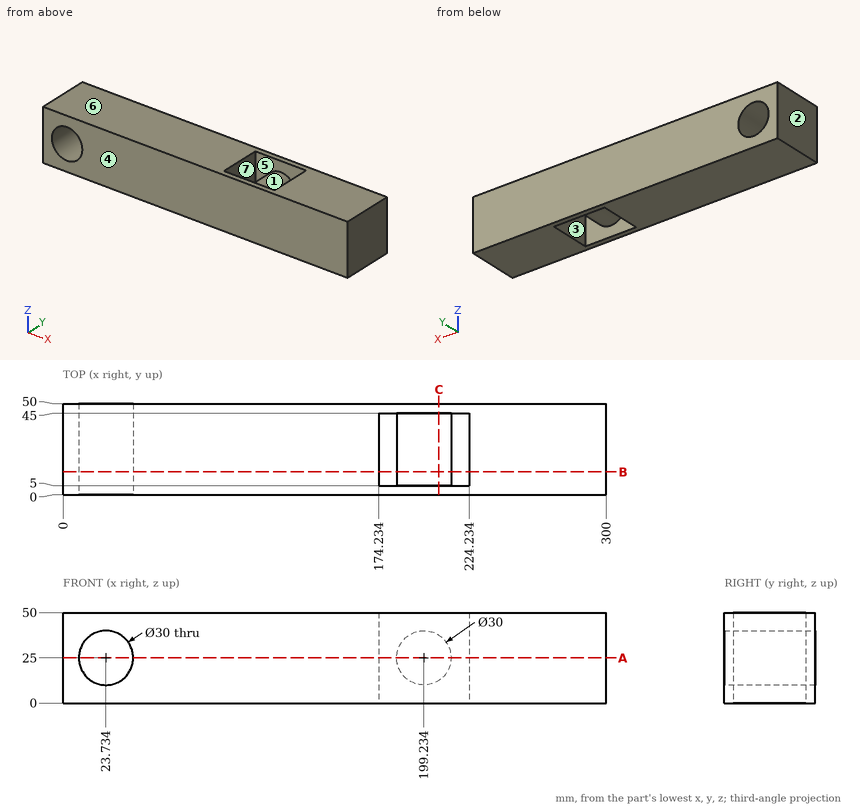
Study the drawing (mm; zero at the part's minimum x, y, z) and answer. A direction names the side the tool comes from. Coordinates: 2 decimals unless noted, no trailing zeros. Loops run counter-clockwise (first coordinate to the right, second up) from the corner with the lowest first, then second, coordinate; pieces in that order, holes last. Notation, with made-up numbers: (65.25, 6) -> (97.25, 6) arc R11 ccw to (97.25, 14) -> close; hole circle Ø11 at (1, 59). An arc over 180 degrees is marked (long way). Write each question's results on one line, items separated by ' | '. Start each with the question number.
1) Find section C-C on x = 207.5. Determine the outline of the cut face in (y, z).
2) Consider line 1 along X through (y, z) = (12.5, 25); line 2 along X through (y, z) = (25.5, 40.5); line 3 along Z through (x, y) = (24.5, 47). Determine where each line is inside the solid, lowest interval first.
3) The mould has two halves that part along Y. Classify the marked faces 4, 5, 6 and 7: pulls with the +Y half, pulls with the -Y half, needs draft (parallel to the pull), parting line crosses it, or undercut.
4) Find section A-A on z = 25. Determine the outline of the cut face in (x, y).
5) Find section B-B on y = 12.5. Determine the outline of the cut face in (x, z), then the cut area to 3 significant figures.
6) For the marked faces 1, 2 and 3, determine the directions among +Z, -Z, +X, -X, +Y, -Y from which every point of the face is accessible in a straight line to the end or side of a thin tool.
Response values:
1) outline: (0, 0) -> (5, 0) -> (5, 12.48) -> (45, 12.48) -> (45, 0) -> (50, 0) -> (50, 50) -> (45, 50) -> (45, 37.52) -> (5, 37.52) -> (5, 50) -> (0, 50) -> close
2) line 1: x = 0 to 8.73, 38.73 to 174.23, 184.23 to 214.23, 224.23 to 300 | line 2: x = 0 to 174.23, 224.23 to 300 | line 3: z = 0 to 10.02, 39.98 to 50
3) face 4: pulls with the -Y half | face 5: undercut | face 6: needs draft | face 7: undercut
4) outline: (0, 0) -> (8.73, 0) -> (8.73, 50) -> (0, 50) -> close; (38.73, 0) -> (300, 0) -> (300, 50) -> (38.73, 50) -> close; hole (174.23, 5) -> (184.23, 5) -> (184.23, 45) -> (174.23, 45) -> close; hole (214.23, 5) -> (224.23, 5) -> (224.23, 45) -> (214.23, 45) -> close
5) outline: (0, 0) -> (174.23, 0) -> (174.23, 50) -> (0, 50) -> close; circle Ø30 at (199.23, 25); (224.23, 0) -> (300, 0) -> (300, 50) -> (224.23, 50) -> close; hole circle Ø30 at (23.73, 25) | area: 12,500 mm^2
6) face 1: none | face 2: +Z, -Z, -X, +Y, -Y | face 3: +Z, -Z
